```python
from build123d import *

# Parameters (mm, degrees)
EXTRUDE_1_DEPTH     = 17
SKETCH_2_R          = 2.5
CUT_EXTRUDE_1_DEPTH = 321.450895562
SKETCH_3_R          = 2.583506321
CUT_EXTRUDE_2_DEPTH = 321.450895562
SKETCH_4_W          = 3.2
SKETCH_4_H          = 25.526459387
SKETCH_4_H_2        = 4
CUT_EXTRUDE_3_DEPTH = 40
SKETCH_5_R          = 2.5
CUT_EXTRUDE_4_DEPTH = 321.450895562
SKETCH_7_W          = 3.2
SKETCH_7_H          = 45
CUT_EXTRUDE_5_DEPTH = 322.082013561
FILLET_1_R          = 5


with BuildPart() as part:
    # 草图1 → 凸台-拉伸1 (new body)
    with BuildSketch(Plane.XY):
        with BuildLine():
            Line((-14.185229692, 14.098909836), (14.185229692, -14.098909836))
            ThreePointArc((14.185229692, -14.098909836), (-14.098909836, -14.185229692), (-14.185229692, 14.098909836))
        make_face()
        Polygon((197.298417852, 226.877355223), (225.668877237, 198.67953555), (14.185229692, -14.098909836), (-14.185229692, 14.098909836), align=None)
        with BuildLine():
            Line((-19.366021875, -4.995717839), (-5.356592379, -19.269325834))
            Line((-5.356592379, -19.269325834), (-21.057561173, -34.67969828))
            ThreePointArc((-21.057561173, -34.67969828), (-26.736053935, -36.969906123), (-32.37077617, -34.57402688))
            Line((-32.37077617, -34.57402688), (-35.172662069, -31.719305281))
            ThreePointArc((-35.172662069, -31.719305281), (-37.462869912, -26.04081252), (-35.06699067, -20.406090285))
            Line((-35.06699067, -20.406090285), (-19.366021875, -4.995717839))
        make_face()
    extrude(amount=EXTRUDE_1_DEPTH)

    # 草图2 → 切除-拉伸1 (cut, through all)
    with BuildSketch(Plane.XY.offset(17)):
        Circle(SKETCH_2_R)
    extrude(amount=-CUT_EXTRUDE_1_DEPTH, mode=Mode.SUBTRACT)

    # 草图3 → 切除-拉伸2 (cut, through all)
    with BuildSketch(Plane.XY.offset(17)):
        with Locations((-21.446298181, -20.977518784)):
            Circle(SKETCH_3_R)
    extrude(amount=-CUT_EXTRUDE_2_DEPTH, mode=Mode.SUBTRACT)

    # 草图4 → 切除-拉伸3 (cut)
    with BuildSketch(Plane(origin=(-33.771719119, -33.146666081, 0), x_dir=(0, 0, 1), z_dir=(-0.7136803997395496, -0.7004714748136406, 0))):
        with Locations((8.5, -14.763229694)):
            Rectangle(SKETCH_4_W, SKETCH_4_H)
        with Locations((8.5, 14.763229694)):
            Rectangle(SKETCH_4_W, SKETCH_4_H)
        with Locations((8.5, 0)):
            Rectangle(SKETCH_4_W, SKETCH_4_H_2)
    extrude(amount=-CUT_EXTRUDE_3_DEPTH, mode=Mode.SUBTRACT)

    # 草图5 → 切除-拉伸4 (cut, through all)
    with BuildSketch(Plane.XY.offset(17)):
        with Locations((21.446298181, 20.977518784)):
            Circle(SKETCH_5_R)
    extrude(amount=-CUT_EXTRUDE_4_DEPTH, mode=Mode.SUBTRACT)

    # 草图7 → 切除-拉伸5 (cut, through all)
    with BuildSketch(Plane(origin=(-14.185229692, 14.098909836, 0), x_dir=(0, 0, 1), z_dir=(-0.7092614846225489, 0.7049454918155146, 0))):
        with Locations((8.5, 29.589308396)):
            Rectangle(SKETCH_7_W, SKETCH_7_H)
    extrude(amount=-CUT_EXTRUDE_5_DEPTH, mode=Mode.SUBTRACT)

    # 圆角1
    fillet_1_edges = [part.edges().sort_by_distance(p)[0] for p in [
        (50.905352818, 22.846030369, 8.5),
        (19.182805686, -9.070736439, 8.5),
        (-9.187653699, 19.127083234, 8.5),
        (22.534893433, 51.043850042, 8.5),
    ]]
    fillet(fillet_1_edges, radius=FILLET_1_R)


solid = part.part
```
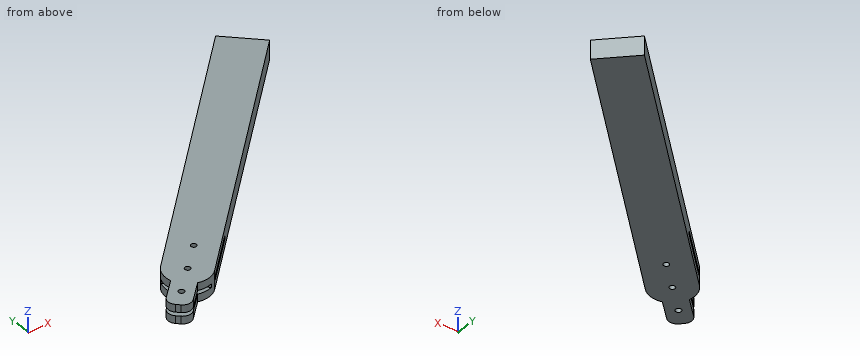
Can you work these out from the model? Positions are in its coordinate system, mm. Round coordinates to 2 decimals unless told otherwise and drop trailing zeros. Loops run counter-clockwise (first coordinate to the right, second up) from the corner with the lowest first, then second, coordinate; pieces in that order, holes last. Notation, with made-up numbers: (21, -34) -> (43, -34) arc R37 ccw to (43, 5) -> close; hole circle Ø11 at (-9, -15.5). An arc over 180 degrees is marked (long way). One line per item, written item: value. Start each with the question number.
1. If I drill on probe 1 along X at (y, z) = (20.5, 11); probe 2 along Y at (x, z) = (0, 6.5); probe 3 along Y at (x, z) = (36.5, 7.25), over which ranges is the centre line in solid material (lowest first)?
2. If we section it at C-C, the plane y = 193.5: Write out the boundary of the cut face in (x, z), then the cut area to 3 significant figures.
3. For pin 1 (10 mm diameter, centred on x = 125.5, z = 2.5, fed in from +Y); pin 2 (5 mm diameter, centred on x = 198, z = 4.5, fed in from -Y); pin 3 (6 mm diameter, centred on y = 146, z = 4, fed in from -X), each with a flat end and sliding along its axis, tell me the tip position at first contact or that it passes through.
4. If we section it at A-A, the plane z = 3.5: Write out the boundary of the cut face in (x, y), then the cut area to 3 significant figures.
5. If we section it at D-D, the plane x = 90.5: Write out the boundary of the cut face in (y, z), then the cut area to 3 significant figures.
6. If we section it at B-B, the plane x = 42: Write out the boundary of the cut face in (y, z), then the cut area to 3 significant figures.
Calculated:
1. probe 1: x = -7.82 to 18.99, 23.9 to 48.57
1. probe 2: y = -20 to -2.5, 2.5 to 28.37
1. probe 3: y = 37.16 to 65.09
2. outline: (164.12, 0) -> (220.52, 0) -> (220.52, 17) -> (164.12, 17) -> close
2. area: 959 mm²
3. pin 1: stops at y = 159.67
3. pin 2: stops at y = 168.33
3. pin 3: stops at x = 113.93
4. outline: (-35.17, -31.72) -> (-32.37, -34.57) arc R8 ccw to (-21.06, -34.68) -> (-5.36, -19.27) arc R20 ccw to (14.19, -14.1) -> (225.67, 198.68) -> (197.3, 226.88) -> (-14.19, 14.1) arc R20 ccw to (-19.37, -5) -> (-35.07, -20.41) arc R8 ccw to start; hole circle Ø5.17 at (-21.45, -20.98); hole circle Ø5 at (0, 0); hole circle Ø5 at (21.45, 20.98)
4. area: 13,100 mm²
5. outline: (62.68, 0) -> (119.43, 0) -> (119.43, 17) -> (62.68, 17) -> close
5. area: 965 mm²
6. outline: (13.89, 0) -> (70.63, 0) -> (70.63, 17) -> (13.89, 17) -> (13.89, 10.1) -> (31.7, 10.1) -> (31.7, 6.9) -> (13.89, 6.9) -> close
6. area: 908 mm²
